Can you work these out from the model? Positions are in its coordinate system, mm. Coordinates: 2 decimals unless noted, no trailing zeros. Loops run counter-clockwise (first coordinate to the right, second up) from the corner with the lowest first, then second, coordinate; pieces in that order, holes last.
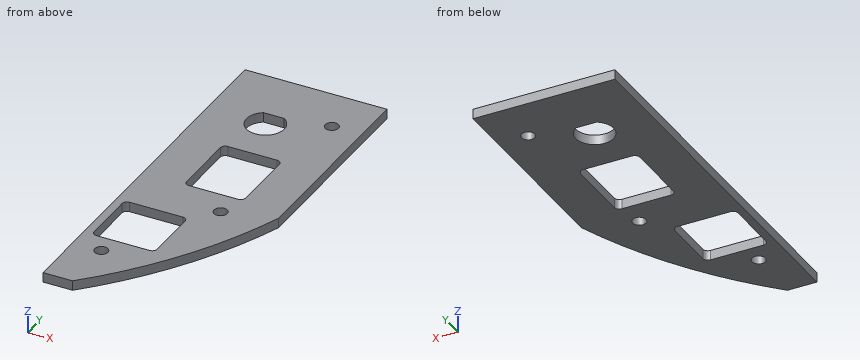
```python
from build123d import *

# Parameters (mm, degrees)
SKETCH1_R             = 1.190050877
BOSS_EXTRUDE1_DEPTH   = 3.175
CUT_EXTRUDE1_DEPTH    = 4.175
SKETCH12_W            = 19.05
SKETCH12_H            = 23.8125
CUT_EXTRUDE2_DEPTH    = 4.175
SKETCH17_W            = 20.32
SKETCH17_H            = 20.32
CUT_EXTRUDE3_DEPTH    = 4.175
FILLET1_R             = 1.5875
F_6_CLEARANCE_HOLE1_D = 4.3053


with BuildPart() as part:
    # Sketch1 → Boss-Extrude1 (new body)
    with BuildSketch(Plane.XY):
        with BuildLine():
            Line((0, -17.78), (0, -141.2875))
            Line((0, -141.2875), (9.525, -141.2875))
            ThreePointArc((9.525, -141.2875), (30.833523511, -114.746148224), (45.72, -84.1375))
            Line((45.72, -84.1375), (45.72, -17.78))
            Line((45.72, -17.78), (0, -17.78))
        make_face()
        with Locations((18.7325, -40.894)):
            Circle(SKETCH1_R, mode=Mode.SUBTRACT)
    extrude(amount=-BOSS_EXTRUDE1_DEPTH)

    # Sketch11 → Cut-Extrude1 (cut, through all)
    with BuildSketch(Plane(origin=(20.844780046, -43.574770805, 0), x_dir=(1, 0, 0), z_dir=(0, 0, 1))):
        with BuildLine():
            Line((-5.443361979, 7.786170805), (1.218801886, 7.786170805))
            ThreePointArc((1.218801886, 7.786170805), (-2.112280046, -3.415229195), (-5.443361979, 7.786170805))
        make_face()
    extrude(amount=-CUT_EXTRUDE1_DEPTH, mode=Mode.SUBTRACT)

    # Sketch12 → Cut-Extrude2 (cut, through all)
    with BuildSketch(Plane.XY):
        with Locations((22.86, -68.54825)):
            Rectangle(SKETCH12_W, SKETCH12_H)
    extrude(amount=-CUT_EXTRUDE2_DEPTH, mode=Mode.SUBTRACT)

    # Sketch17 → Cut-Extrude3 (cut, through all)
    with BuildSketch(Plane.XY):
        with Locations((12.731722108, -106.422544949)):
            Rectangle(SKETCH17_W, SKETCH17_H)
    extrude(amount=-CUT_EXTRUDE3_DEPTH, mode=Mode.SUBTRACT)

    # Fillet1
    fillet1_edges = [part.edges().sort_by_distance(p)[0] for p in [
        (13.335, -80.4545, -1.5875),
        (13.335, -56.642, -1.5875),
        (32.385, -56.642, -1.5875),
        (32.385, -80.4545, -1.5875),
        (22.891722108, -96.262544949, -1.5875),
        (22.891722108, -116.582544949, -1.5875),
        (2.571722108, -116.582544949, -1.5875),
        (2.571722108, -96.262544949, -1.5875),
    ]]
    fillet(fillet1_edges, radius=FILLET1_R)

    # #6 Clearance Hole1 (through all)
    with Locations(Plane.XY):
        with Locations((9.144, -122.9995), (29.5275, -88.7095), (36.1315, -33.274)):
            Hole(F_6_CLEARANCE_HOLE1_D / 2)


solid = part.part
```
Item 1: Suppose I cut it at C-C, the plane x = 29.5. Please give me the cut outline in (y, z) (1 decimal), plus the area to 3 significant figures.
Results are:
outline: (-116.8, -3.2) - (-90.9, -3.2) - (-90.9, 0) - (-116.8, 0) - close; (-86.6, -3.2) - (-80.5, -3.2) - (-80.5, 0) - (-86.6, 0) - close; (-56.6, -3.2) - (-17.8, -3.2) - (-17.8, 0) - (-56.6, 0) - close
area: 225 mm2
Item 2: I need wall thicknesses on line 1 along Y through (x, z) = (23.5, -2.6); line 2 along X through (y, z) = (-64, -2.3) (3 decimals); line 3 along X through (y, z) = (-58, -2.9). Which ranges of each line are inside material? Lowest first, please.
Results are:
line 1: y = -125.31 to -80.45, -56.64 to -44.69, -37.1 to -17.78
line 2: x = 0 to 13.335, 32.385 to 45.72
line 3: x = 0 to 13.35, 32.37 to 45.72
Item 3: I'm going to push flat-ended pins straight in: P1, Ø1, axis at x = 35.5, y = -58, coming from the +Z side; P2, Ø3.5, axis at x = 9.14, y = -123, coming from the +Z side; P3, Ø1.6, axis at x = 17.5, z = -2.5, coming from the -Y side. Where does each tip first touch, or does it pass through?
Results are:
P1: stops at z = 0
P2: passes through
P3: stops at y = -133.65
Item 4: Suppose I cut it at A-A, the plane x = 17.5. Please give me the cut outline in (y, z) (1 decimal).
Results are:
outline: (-132.7, -3.2) - (-116.6, -3.2) - (-116.6, 0) - (-132.7, 0) - close; (-96.3, -3.2) - (-80.5, -3.2) - (-80.5, 0) - (-96.3, 0) - close; (-56.6, -3.2) - (-46.9, -3.2) - (-46.9, 0) - (-56.6, 0) - close; (-35.8, -3.2) - (-17.8, -3.2) - (-17.8, 0) - (-35.8, 0) - close
Item 5: Suppose I cut it at D-D, the plane z = -0.7. Please give me the cut outline in (x, y) (1 decimal).
Results are:
outline: (0, -141.3) - (9.5, -141.3) arc R152.4 ccw to (45.7, -84.1) - (45.7, -17.8) - (0, -17.8) - close; hole (2.6, -115) arc R1.6 ccw to (4.2, -116.6) - (21.3, -116.6) arc R1.6 ccw to (22.9, -115) - (22.9, -97.9) arc R1.6 ccw to (21.3, -96.3) - (4.2, -96.3) arc R1.6 ccw to (2.6, -97.9) - close; hole circle Ø4.3 at (9.1, -123); hole (13.3, -78.9) arc R1.6 ccw to (14.9, -80.5) - (30.8, -80.5) arc R1.6 ccw to (32.4, -78.9) - (32.4, -58.2) arc R1.6 ccw to (30.8, -56.6) - (14.9, -56.6) arc R1.6 ccw to (13.3, -58.2) - close; hole (15.4, -35.8) arc R6.1 ccw (long way) to (22.1, -35.8) - close; hole circle Ø4.3 at (29.5, -88.7); hole circle Ø4.3 at (36.1, -33.3)
Item 6: Suppose I cut it at B-B, the plane y = -103. Please give me the cut outline in (x, z) (3 decimals), plus the area to 3 significant figures.
Results are:
outline: (0, -3.175) - (2.572, -3.175) - (2.572, 0) - (0, 0) - close; (22.892, -3.175) - (37.561, -3.175) - (37.561, 0) - (22.892, 0) - close
area: 54.7 mm2
